from build123d import *

# Parameters (mm, degrees)
SKETCH2_W                                       = 30
SKETCH2_H                                       = 20
BOSS_EXTRUDE1_DEPTH                             = 25
SKETCH3_W                                       = 83
SKETCH3_H                                       = 50
BOSS_EXTRUDE2_DEPTH                             = 10
CSK_FOR_M4_FLAT_HEAD_MACHINE_SCREW1_D           = 4.5
CSK_FOR_M4_FLAT_HEAD_MACHINE_SCREW1_CSINK_D     = 13.4
CSK_FOR_M4_FLAT_HEAD_MACHINE_SCREW1_CSINK_ANGLE = 90
FILLET1_R                                       = 10
FILLET2_R                                       = 10
FILLET3_R                                       = 3


with BuildPart() as part:
    # Sketch2 → Boss-Extrude1 (new body)
    with BuildSketch(Plane.XY):
        with Locations((-28.360190379, 6.518738069)):
            Rectangle(SKETCH2_W, SKETCH2_H)
    extrude(amount=BOSS_EXTRUDE1_DEPTH)

    # Sketch3 → Boss-Extrude2 (add)
    with BuildSketch(Plane.XY.offset(25)):
        with Locations((-1.860190379, 6.518738069)):
            Rectangle(SKETCH3_W, SKETCH3_H)
    extrude(amount=-BOSS_EXTRUDE2_DEPTH)

    # CSK for M4 Flat Head Machine Screw1 (through all)
    with Locations(Plane.XY.offset(25)):
        with Locations((-35.714941389, 6.421876295), (-20.714941389, 6.421876295)):
            CounterSinkHole(CSK_FOR_M4_FLAT_HEAD_MACHINE_SCREW1_D / 2, CSK_FOR_M4_FLAT_HEAD_MACHINE_SCREW1_CSINK_D / 2, counter_sink_angle=CSK_FOR_M4_FLAT_HEAD_MACHINE_SCREW1_CSINK_ANGLE)

    # Fillet1
    fillet1_edges = [part.edges().sort_by_distance(p)[0] for p in [
        (-43.360190379, -18.481261931, 20),
        (-43.360190379, 31.518738069, 20),
        (39.639809621, 31.518738069, 20),
        (39.639809621, -18.481261931, 20),
    ]]
    fillet(fillet1_edges, radius=FILLET1_R)

    # Fillet2
    fillet2_edges = [part.edges().sort_by_distance(p)[0] for p in [
        (-28.360190379, -3.481261931, 15),
        (-13.360190379, 6.518738069, 15),
        (-28.360190379, 16.518738069, 15),
    ]]
    fillet(fillet2_edges, radius=FILLET2_R)

    # Fillet3
    fillet3_edges = [part.edges().sort_by_distance(p)[0] for p in [
        (-28.360190379, -3.481261931, 0),
        (-13.360190379, 6.518738069, 0),
        (-28.360190379, 16.518738069, 0),
        (-43.360190379, 6.518738069, 0),
    ]]
    fillet(fillet3_edges, radius=FILLET3_R)


solid = part.part
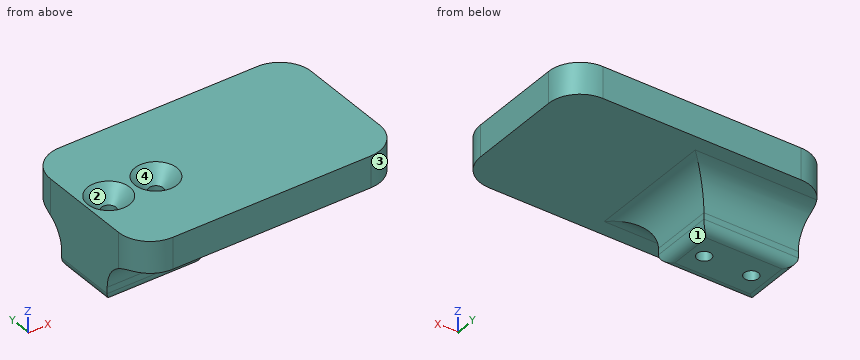
The listing builds one solid part. Answer for the finished solid, in the listing's coordinates (mm). Face numbers are marked on the shaded views. Round coordinates to 2 decimals unless told otherwise and drop trailing zeros. Write each loop counter-clockwise with the first axis right and the second up, starting at its lowest first coordinate (ties: lowest second). Pieces come first, ordered by that corner, then holes. Notation, with made-up numbers: M -4,-10 L 10,-10 A13 ccw 10,-4 Z; hole C -36.75,9 d5. An arc over 180 degrees is marked long. Write each question's results on one line, items separated by ' | '. Start each with the question number.
Item 1: Find section D-D on z = 22.75. Write down the section's boundary in (x, y), and give its area (3 significant figures).
Item 2: Straight lines are drawn through the part: probe 1 along X at (y, z) = (9, 23.5); probe 2 along X at (y, z) = (7, 23.5); probe 3 along Z at (x, y) = (22, 5.5). For each, find the intervals that lie inside material, in ascending order.
Item 3: Given pin 1 Ø1.6 at (x, z) = (-27, 4) entering from -Y; pin 2 Ø1 at (y, z) = (10.5, 4) entering from +X; pin 3 Ø1.6 at (x, z) = (-34.5, 4.5) entering from +Y, each flat-ended and moving along its own axis, determine where each tip first touches the part or whether it passes through.
Item 4: Find section C-C on y = -6.5. Write down the section's boundary in (x, z).
Item 5: Find section B-B on x = -9.5. Write down the section's boundary in (y, z).
Item 6: Find section A-A on z = 16. Write down the section's boundary in (x, y).
Item 7: The mould has two halves that part along Y. Classify the marked faces 1, 2, 3 and 4: +Y half, -Y half, draft (parallel to the pull), parting line (faces both ways), or undercut.
Answer block:
1) outline: M -43.36,-8.48 A10 ccw -33.36,-18.48 L 29.64,-18.48 A10 ccw 39.64,-8.48 L 39.64,21.52 A10 ccw 29.64,31.52 L -33.36,31.52 A10 ccw -43.36,21.52 Z; hole C -35.71,6.42 d8.9; hole C -20.71,6.42 d8.9 | area: 3,940 mm²
2) probe 1: x = -43.36 to -40.23, -31.2 to -25.23, -16.2 to 39.64 | probe 2: x = -43.36 to -40.88, -30.55 to -25.88, -15.55 to 39.64 | probe 3: z = 15 to 25
3) pin 1: stops at y = -3.48 | pin 2: stops at x = -13.36 | pin 3: stops at y = 16.52
4) outline: M -43.36,12.16 L -10.34,12.16 A10 cw -3.36,15 L 39.64,15 L 39.64,25 L -43.36,25 Z
5) outline: M -18.48,15 L -13.48,15 A10 cw -7.34,12.89 L 20.38,12.89 A10 cw 26.52,15 L 31.52,15 L 31.52,25 L -18.48,25 Z
6) outline: M -43.36,-8.48 A10 ccw -33.36,-18.48 L 29.64,-18.48 A10 ccw 39.64,-8.48 L 39.64,21.52 A10 ccw 29.64,31.52 L -33.36,31.52 A10 ccw -43.36,21.52 Z; hole C -35.71,6.42 d4.5; hole C -20.71,6.42 d4.5
7) face 1: draft | face 2: undercut | face 3: -Y half | face 4: undercut
